```python
from build123d import *

# Parameters (mm, degrees)
SKETCH1_W           = 152.4
SKETCH1_H           = 38.1
SKETCH1_R           = 4.1656
BOSS_EXTRUDE1_DEPTH = 3.175


with BuildPart() as part:
    # Sketch1 → Boss-Extrude1 (new, symmetric)
    with BuildSketch(Plane.XY):
        with Locations((76.2, 19.05)):
            Rectangle(SKETCH1_W, SKETCH1_H)
        with Locations((19.05, 19.05)):
            Circle(SKETCH1_R, mode=Mode.SUBTRACT)
        with Locations((57.15, 19.05)):
            Circle(SKETCH1_R, mode=Mode.SUBTRACT)
        with Locations((95.25, 19.05)):
            Circle(SKETCH1_R, mode=Mode.SUBTRACT)
        with Locations((133.35, 19.05)):
            Circle(SKETCH1_R, mode=Mode.SUBTRACT)
    extrude(amount=BOSS_EXTRUDE1_DEPTH, both=True)


solid = part.part
```
The listing builds one solid part. Answer for the finished solid, in the listing's coordinates (mm). Give positions to 0.01 mm unless a question says otherwise; leave off trailing zeros. Order: outer loops, then holes, each group sorted by start corner. A loop starts at its lowest first (then second) coordinate and runs counter-clockwise, first axis right, second up.
1) Consider line 1 along X through (y, z) = (19.5, 2); line 2 along Y through (x, z) = (133.35, 0.5); line 3 along X through (y, z) = (20, 1). Determine where each line is inside the solid, lowest interval first.
Reported:
line 1: x = 0 to 14.91, 23.19 to 53.01, 61.29 to 91.11, 99.39 to 129.21, 137.49 to 152.4
line 2: y = 0 to 14.88, 23.22 to 38.1
line 3: x = 0 to 14.99, 23.11 to 53.09, 61.21 to 91.19, 99.31 to 129.29, 137.41 to 152.4
2) Given P1, Ø6.5, axis at x = 133.35, y = 19.05, coming from the +Z side, flat-ended and moving along its own axis, determine where the tip first touches the part or whether it passes through.
Reported:
P1: passes through
3) Find section A-A on y = 19.05. Write down the section's boundary in (x, z) (3 decimals).
Reported:
outline: (0, -3.175) - (14.884, -3.175) - (14.884, 3.175) - (0, 3.175) - close; (23.216, -3.175) - (52.984, -3.175) - (52.984, 3.175) - (23.216, 3.175) - close; (61.316, -3.175) - (91.084, -3.175) - (91.084, 3.175) - (61.316, 3.175) - close; (99.416, -3.175) - (129.184, -3.175) - (129.184, 3.175) - (99.416, 3.175) - close; (137.516, -3.175) - (152.4, -3.175) - (152.4, 3.175) - (137.516, 3.175) - close
4) Find section C-C on z = 0. Write down the section's boundary in (x, y).
Reported:
outline: (0, 0) - (152.4, 0) - (152.4, 38.1) - (0, 38.1) - close; hole circle Ø8.33 at (19.05, 19.05); hole circle Ø8.33 at (57.15, 19.05); hole circle Ø8.33 at (95.25, 19.05); hole circle Ø8.33 at (133.35, 19.05)
5) Find section B-B on x = 133.35. Write down the section's boundary in (y, z) (3 decimals).
Reported:
outline: (0, -3.175) - (14.884, -3.175) - (14.884, 3.175) - (0, 3.175) - close; (23.216, -3.175) - (38.1, -3.175) - (38.1, 3.175) - (23.216, 3.175) - close
6) Determine the mould class of faces 1 (the face through (75, 0, 0)), 2 (the face through (152.4, 19, 0)), 3 (the face through (53.84, 16.52, -0.04)) for opening direction X: pulls with the +X half, pulls with the -X half, needs draft (parallel to the pull), parting line crosses it, or undercut.
Reported:
face 1: needs draft
face 2: pulls with the +X half
face 3: undercut
7) Find section D-D on x = 96.5. Write down the section's boundary in (y, z) (3 decimals).
Reported:
outline: (0, -3.175) - (15.076, -3.175) - (15.076, 3.175) - (0, 3.175) - close; (23.024, -3.175) - (38.1, -3.175) - (38.1, 3.175) - (23.024, 3.175) - close
